The listing builds one solid part. Answer for the finished solid, in the listing's coordinates (mm). Face numbers are marked on the shaded views. A direction names the side the tool comes from. Give positions to 0.01 mm unless a question says otherwise; leave off trailing zeros. Order: outer loops, then holes, each group sorted by start corner. A loop starts at its lowest first (then second) coordinate and runs counter-clockwise, first axis right, second up. Notation, with made-up numbers: (-10.75, -28.5) - (12.25, -28.5) arc R32 ccw to (12.25, 0.5) - close; hole circle Ø10 at (70.5, 8). An arc over 180 degrees is marked (long way). Write each question's results on one line, items separated by ' | '. Start each with the question number.
1. Find the intervals of material crossed by L1, parallel to Z at x = 6.5, y = 10; L2, parallel to Y at x = 29.35, z = 0; L3, parallel to Y at x = 37.5, z = -23.75, in increasing order.
2. Section B-B (y = 4) is taken. Give the vertices of the cut face in (x, z), and give its area (3 significant figures).
3. Which of the six approach directions +Z, -Z, +X, -X, +Y, -Y give full straight-line access (tool end or side, diameter ignored) to the marked faces 1, 2, 3, 4 and 5?
4. Determine the mould class of the marked faces 6, 7 and 8 for opening direction Z: released by +Z, released by -Z, zero draft, split by the parting line, or undercut.
5. Flat-ended cylindrical pins translate along their axes: pin 1 (3 mm diameter, centred on y = 30, z = -3.5, fed in from -X); pin 2 (3 mm diameter, centred on x = 7.83, y = 29.59, fed in from -Z); pin 3 (4 mm diameter, centred on x = 22.55, y = 17.57, fed in from +Z). Find the tip coordinate at first contact, or state that the pin passes through.
6. Section A-A (z = 0) is taken. Give the vertices of the cut face in (x, y), and give its area (3 significant figures).
7. Section D-D (x = 13) is taken. Give the vertices of the cut face in (y, z), and give its area (3 significant figures).
8. Section C-C (x = 0) is taken. Give the vertices of the cut face in (y, z).
from build123d import *

# Parameters (mm, degrees)
BOSS_EXTRUDE1_DEPTH      = 30
BOSS_EXTRUDE1_DEPTH_BACK = 30
SKETCH2_R                = 3.25
SKETCH2_R_2              = 1.25
SKETCH2_R_3              = 5
SKETCH3_W                = 72
SKETCH3_H                = 55
CUT_EXTRUDE1_DEPTH       = 56.8323383
SKETCH4_W                = 10
SKETCH4_H                = 8
BOSS_EXTRUDE2_DEPTH      = 10
FILLET1_R                = 4
SKETCH5_R                = 1.75
CUT_EXTRUDE2_DEPTH       = 74.805487601
FILLET1_OF_MIRROR1_R     = 4
FILLET2_R                = 4
SKETCH6_R                = 1.25
SKETCH6_R_2              = 5
BOSS_EXTRUDE3_DEPTH      = 3
SKETCH7_R                = 2.5
CUT_EXTRUDE3_DEPTH       = 2
SKETCH8_R                = 2
CUT_EXTRUDE4_DEPTH       = 59.489315264


with BuildPart() as part:
    # Sketch2 → Boss-Extrude1 (new, two sides: drawn at the far end of the back side and taken through both)
    with BuildSketch(Plane.XY.offset(-BOSS_EXTRUDE1_DEPTH_BACK)):
        with BuildLine():
            Line((-7.5, 5), (-7.5, 15))
            Line((-7.5, 15), (9.281992624, 35))
            Line((9.281992624, 35), (31.5, 35))
            Line((31.5, 35), (31.5, 10))
            Line((31.5, 10), (7.5, 10))
            Line((7.5, 10), (7.5, 5))
            ThreePointArc((7.5, 5), (6.035533906, 1.464466094), (2.5, 0))
            Line((2.5, 0), (-2.5, 0))
            ThreePointArc((-2.5, 0), (-6.035533906, 1.464466094), (-7.5, 5))
        make_face()
        with Locations((0, 5)):
            Circle(SKETCH2_R, mode=Mode.SUBTRACT)
        with Locations((22.545074696, 17.568596061)):
            Circle(SKETCH2_R_2, mode=Mode.SUBTRACT)
        with Locations((7.834882147, 29.593995644)):
            Circle(SKETCH2_R_2, mode=Mode.SUBTRACT)
        with Locations((13.291231119, 21.258633871)):
            Circle(SKETCH2_R_3, mode=Mode.SUBTRACT)
    extrude(amount=BOSS_EXTRUDE1_DEPTH + BOSS_EXTRUDE1_DEPTH_BACK)

    # Sketch3 → Cut-Extrude1 (cut, through all)
    with BuildSketch(Plane(origin=(0, 35, 0), x_dir=(1, 0, 0), z_dir=(0, 1, 0))):
        with Locations((-7.5, 0)):
            Rectangle(SKETCH3_W, SKETCH3_H)
    extrude(amount=-CUT_EXTRUDE1_DEPTH, mode=Mode.SUBTRACT)

    # Sketch4 → Boss-Extrude2 (add)
    with BuildSketch(Plane(origin=(31.5, 0, 0), x_dir=(0, 0, -1), z_dir=(1, 0, 0))):
        with Locations((-25, 31)):
            Rectangle(SKETCH4_W, SKETCH4_H)
    boss_extrude2 = extrude(amount=BOSS_EXTRUDE2_DEPTH)

    # Fillet1
    fillet1_edges = [part.edges().sort_by_distance(p)[0] for p in [
        (41.5, 27, 25),
        (41.5, 35, 25),
    ]]
    fillet(fillet1_edges, radius=FILLET1_R - 0.0001)  # a hair under: the kernel refuses the full size

    # Sketch5 → Cut-Extrude2 (cut, through all)
    with BuildSketch(Plane(origin=(0, 0, 20), x_dir=(-1, 0, 0), z_dir=(0, 0, -1))):
        with Locations((-37.5, 31)):
            Circle(SKETCH5_R)
    cut_extrude2 = extrude(amount=-CUT_EXTRUDE2_DEPTH, mode=Mode.SUBTRACT)

    # Mirror1: Boss-Extrude2, Cut-Extrude2 across plane
    add(boss_extrude2.mirror(Plane.XY))
    add(cut_extrude2.mirror(Plane.XY), mode=Mode.SUBTRACT)

    # Fillet1 of Mirror1
    fillet1_of_mirror1_edges = [part.edges().sort_by_distance(p)[0] for p in [
        (41.5, 27, -25),
        (41.5, 35, -25),
    ]]
    fillet(fillet1_of_mirror1_edges, radius=FILLET1_OF_MIRROR1_R - 0.0001)  # a hair under: the kernel refuses the full size

    # Fillet2
    fillet2_edges = [part.edges().sort_by_distance(p)[0] for p in [
        (31.5, 27, 25),
        (31.5, 31, 20),
        (31.5, 27, -25),
        (31.5, 31, -20),
        (9.281992624, 35, -28.75),
        (7.5, 10, -28.75),
        (-7.5, 15, -28.75),
        (-7.5, 15, 28.75),
        (7.5, 10, 28.75),
        (9.281992624, 35, 28.75),
    ]]
    fillet(fillet2_edges, radius=FILLET2_R)

    # Sketch6 → Boss-Extrude3 (add)
    with BuildSketch(Plane.XY.offset(-27.5)):
        with BuildLine():
            Line((28.5, 35), (11.147223256, 35))
            ThreePointArc((11.147223256, 35), (9.456750209, 34.625231148), (8.083045484, 33.571150439))
            Line((8.083045484, 33.571150439), (-6.564177772, 16.115269502))
            ThreePointArc((-6.564177772, 16.115269502), (3.098200373, 14.919475381), (11.5, 10))
            Line((11.5, 10), (28.5, 10))
            Line((28.5, 10), (28.5, 35))
        make_face()
        with Locations((22.545074696, 17.568596061)):
            Circle(SKETCH6_R, mode=Mode.SUBTRACT)
        with Locations((13.291231119, 21.258633871)):
            Circle(SKETCH6_R_2, mode=Mode.SUBTRACT)
        with Locations((7.834882147, 29.593995644)):
            Circle(SKETCH6_R, mode=Mode.SUBTRACT)
    boss_extrude3 = extrude(amount=BOSS_EXTRUDE3_DEPTH)

    # Sketch7 → Cut-Extrude3 (cut)
    with BuildSketch(Plane(origin=(0, 0, -30), x_dir=(-1, 0, 0), z_dir=(0, 0, -1))):
        with Locations((-22.545074696, 17.568596061)):
            Circle(SKETCH7_R)
        with Locations((-7.834882147, 29.593995644)):
            Circle(SKETCH7_R)
    cut_extrude3 = extrude(amount=-CUT_EXTRUDE3_DEPTH, mode=Mode.SUBTRACT)

    # Mirror2: Boss-Extrude3, Cut-Extrude3 across plane
    add(boss_extrude3.mirror(Plane.XY))
    add(cut_extrude3.mirror(Plane.XY), mode=Mode.SUBTRACT)

    # Sketch8 → Cut-Extrude4 (cut, through all)
    with BuildSketch(Plane.ZY.offset(-28.5)):
        with Locations((0, 16)):
            Circle(SKETCH8_R)
    extrude(amount=-CUT_EXTRUDE4_DEPTH, mode=Mode.SUBTRACT)


solid = part.part
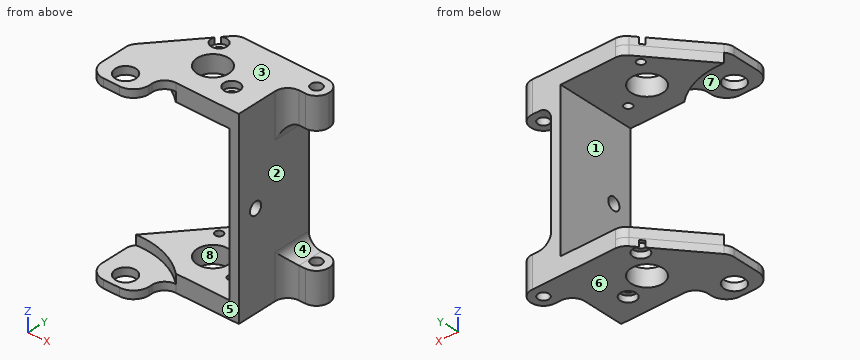
Reported:
1) L1: -30 to -27.5, 27.5 to 30 | L2: 10 to 14, 18 to 35 | L3: 27 to 29.25, 32.75 to 35
2) outline: (-7.4, -30) - (-3.09, -30) - (-3.09, -27.5) - (-7.4, -27.5) - close; (-7.4, 27.5) - (-3.09, 27.5) - (-3.09, 30) - (-7.4, 30) - close; (3.09, -30) - (7.4, -30) - (7.4, -27.5) - (3.09, -27.5) - close; (3.09, 27.5) - (7.4, 27.5) - (7.4, 30) - (3.09, 30) - close | area: 43.1 mm²
3) face 1: -X, +Y, -Y | face 2: +X, -Y | face 3: +Z, +X, -X, +Y, -Y | face 4: +X, +Y, -Y | face 5: +Z, -Z, +X, -Y
4) face 6: released by -Z | face 7: undercut | face 8: zero draft
5) pin 1: x = 28.5 | pin 2: z = -28 | pin 3: z = 28
6) outline: (28.5, 10) - (31.5, 10) - (31.5, 14) - (28.5, 14) - close; (28.5, 18) - (31.5, 18) - (31.5, 35) - (28.5, 35) - close | area: 63.0 mm²
7) outline: (10, -30) - (16.27, -30) - (16.27, -24.5) - (10, -24.5) - close; (10, 24.5) - (16.27, 24.5) - (16.27, 30) - (10, 30) - close; (26.25, -30) - (35, -30) - (35, -24.5) - (26.25, -24.5) - close; (26.25, 24.5) - (35, 24.5) - (35, 30) - (26.25, 30) - close | area: 165 mm²
8) outline: (0, -30) - (1.75, -30) - (1.75, -27.5) - (0, -27.5) - close; (0, 27.5) - (1.75, 27.5) - (1.75, 30) - (0, 30) - close; (8.25, -30) - (23.94, -30) - (23.94, -24.5) - (15.74, -24.5) - (15.74, -27.5) - (8.25, -27.5) - close; (8.25, 27.5) - (15.74, 27.5) - (15.74, 24.5) - (23.94, 24.5) - (23.94, 30) - (8.25, 30) - close
